Autodesk Inventor part; units mm, degrees
ref_plane "YZ Plane" through (0, 0, 0) normal (1, 0, 0) x (0, 1, 0)
ref_plane "XZ Plane" through (0, 0, 0) normal (0, 1, 0) x (-1, 0, 0)
ref_plane "XY Plane" through (0, 0, 0) normal (0, 0, 1) x (1, 0, 0)
sketch "Sketch1" plane through (0, 0, 0) normal (0, 1, 0) x (-1, 0, 0)
  circle A0 centre (0, 0) radius 50
  dimension "d0" = 100
extrude "Extrusion1" add sketch "Sketch1" along normal mid plane 5
sketch "Sketch2" plane through (0, 2.5, 0) normal (0, 1, 0) x (1, 0, 0)
  line L0 (-5, 5) -> (5, 5) construction
  line L1 (5, 5) -> (5, -5) construction
  line L2 (5, -5) -> (-5, -5) construction
  line L3 (-5, -5) -> (-5, 5) construction
  line L4 (-5, 5) -> (5, -5) construction
  line L5 (5, 5) -> (-5, -5) construction
  circle A0 centre (5, 5) radius 2.75
  circle A1 centre (-5, -5) radius 2.75
  point P0 (0, 0)
  dimension "d77" = 10
  dimension "d78" = 10
  dimension "d80" = 5.5
  dimension "d81" = 5.5
extrude "Extrusion2" cut sketch "Sketch2" against normal blind 10
sketch "Sketch3" plane through (0, 2.5, 0) normal (0, 1, 0) x (1, 0, 0)
  line L0 (0, 0) -> (25, 0) construction
  line L1 (18.8, -11.3) -> (31.2, -11.3)
  line L2 (31.2, -11.3) -> (31.2, 11.3)
  line L3 (31.2, 11.3) -> (18.8, 11.3)
  line L4 (18.8, 11.3) -> (18.8, -11.3)
  line L5 (18.8, -11.3) -> (31.2, 11.3) construction
  line L6 (31.2, -11.3) -> (18.8, 11.3) construction
  line L7 (25, 0) -> (25, 14.25) construction
  line L8 (25, 0) -> (25, -14.25) construction
  circle A0 centre (25, 14.25) radius 1.1
  circle A1 centre (25, -14.25) radius 1.1
  dimension "d9" = 25
  dimension "d10" = 12.4
  dimension "d11" = 22.6
  dimension "d21" = 14.25
  dimension "d22" = 14.25
  dimension "d23" = 2.2
  dimension "d24" = 2.2
extrude "Extrusion3" cut sketch "Sketch3" against normal blind 10
sketch "Sketch5" plane through (0, -2.5, 0) normal (0, -1, 0) x (1, 0, 0)
  line L0 (31.2, -11.3) -> (33.7, -11.3)
  line L1 (33.7, -11.3) -> (33.7, 11.3)
  line L2 (33.7, 11.3) -> (31.2, 11.3)
  line L3 (31.2, 11.3) -> (31.2, -11.3)
  line L4 (31.2, -11.3) -> (31.2, 11.3) construction
  line L5 (31.2, 0) -> (39.7, 0) construction
  line L6 (39.7, 0) -> (39.7, -20) construction
  line L7 (39.7, -20) -> (31.2, -20)
  line L8 (31.2, -20) -> (31.2, 20)
  line L9 (31.2, 20) -> (39.7, 20)
  line L10 (39.7, 20) -> (39.7, -20)
  line L11 (33.7, -11.3) -> (33.7, -20)
  line L12 (33.7, 11.3) -> (33.7, 20)
  point P0 (0, 0)
  point P1 (31.2, 11.3)
  dimension "d34" = 2.5
  dimension "d35" = 8.5
  dimension "d36" = 20
  dimension "d37" = 40
extrude "Extrusion5" add sketch "Sketch5" along normal blind 11.8 contours L1 L12 L9 L10 L7 L11
sketch "Sketch6" plane through (0, -2.5, 0) normal (0, -1, 0) x (1, 0, 0)
  line L0 (31.2, -11.3) -> (31.2, 11.3)
  line L1 (31.2, 0) -> (33.7, 0)
  line L2 (33.7, 0) -> (33.7, -20)
  line L3 (33.7, -20) -> (31.2, -20)
  line L4 (31.2, -20) -> (31.2, 0)
  line L5 (39.7, 20) -> (33.7, 20)
  line L6 (31.2, 0) -> (33.7, 0)
  line L7 (33.7, 0) -> (33.7, 20)
  line L8 (33.7, 20) -> (31.2, 20)
  line L9 (31.2, 20) -> (31.2, 0)
  line L10 (18.8, 11.3) -> (31.2, 11.3)
  line L11 (31.2, 11.3) -> (33.7, 11.3)
  line L12 (33.7, -20) -> (33.7, 20)
  line L13 (39.7, 20) -> (42.2, 20)
  line L14 (42.2, 20) -> (42.2, -20)
  line L15 (42.2, -20) -> (39.7, -20)
  line L16 (39.7, -20) -> (39.7, 20)
  line L17 (31.2, -15.9678) -> (33.7, -15.9678)
  point P0 (0, 0)
  point P1 (31.2, 11.3)
  dimension "d40" = 2.5
extrude "Extrusion6" add sketch "Sketch6" along normal blind 16.8 contours L13 L14 L15 L16 | L17 L2 L3 L4 | L9 L8 L7 L11
sketch "Sketch7" plane through (0, -19.3, 0) normal (0, -1, 0) x (1, 0, 0)
  line L0 (42.2, -20) -> (31.2, -20)
  line L1 (31.2, -20) -> (42.2, -20)
  line L2 (42.2, -20) -> (42.2, 0)
  line L3 (42.2, 0) -> (31.2, 0)
  line L4 (31.2, 0) -> (31.2, -20)
  point P0 (0, 0)
extrude "Extrusion7" add sketch "Sketch7" along normal blind 2.5
sketch "Sketch8" plane through (31.2, -19.3, 0) normal (0, 0, 1) x (1, 0, 0)
  line L0 (0, -2.5) -> (11, -2.5) construction
  line L1 (5.5, -2.5) -> (5.5, -10) construction
  circle A0 centre (5.5, -10) radius 7.5
  line L2 (0, 16.8) -> (0, -2.5) construction
  line L3 (11, 16.8) -> (11, -2.5)
  line L4 (11, -2.5) -> (11, -4.901)
  line L5 (0, -2.5) -> (0, -4.901)
  line L6 (11, -2.5) -> (0, -2.5)
  point P0 (-31.2, 19.3)
  dimension "d45" = 7.5
extrude "Extrusion8" add sketch "Sketch8" against normal blind 3
fillet "Fillet1" radius 8.25 1 edges at (36.7, -21.8, -3)
sketch "Sketch9" plane through (42.2, -2.5, -20) normal (0, 0, -1) x (-1, 0, 0)
  line L0 (11, -16.8) -> (8.5, -16.8)
  line L1 (8.5, -16.8) -> (2.5, -16.8)
  line L2 (2.5, -16.8) -> (2.5, -11.8)
  line L3 (2.5, -11.8) -> (8.5, -11.8)
  line L4 (8.5, -11.8) -> (8.5, -16.8)
  line L5 (11, 0) -> (11, -19.3)
  line L6 (0, 0) -> (0, -19.3)
  line L7 (11, -19.3) -> (0, -19.3)
  line L8 (0, -19.3) -> (0, -9.35)
  line L9 (0, -9.35) -> (11, -9.35)
  line L10 (11, -9.35) -> (11, -19.3)
  point P0 (42.2, 2.5)
  dimension "d49" = 9.95
extrude "Extrusion9" add sketch "Sketch9" along normal blind 10
sketch "Sketch12" plane through (0, 2.5, 0) normal (0, 1, 0) x (1, 0, 0)
  circle A0 centre (-25, 0) radius 12.5 construction
  line L0 (-25, 0) -> (-18.75, -10.8253) construction
  line L1 (-25, 0) -> (-37.5, 0) construction
  line L2 (-25, 0) -> (-18.75, 10.8253) construction
  circle A1 centre (-37.5, 0) radius 2.75
  circle A2 centre (-18.75, 10.8253) radius 2.75
  circle A3 centre (-18.75, -10.8253) radius 2.75
  point P0 (0, 0)
  dimension "d64" = 25
  dimension "d65" = 120
  dimension "d67" = 5.5
  dimension "d68" = 5.5
  dimension "d69" = 5.5
  dimension "d70" = 25
extrude "Extrusion12" cut sketch "Sketch12" against normal blind 10
sketch "Sketch13" plane through (0, -2.5, 0) normal (0, -1, 0) x (1, 0, 0)
  line L0 (0, 0) -> (0, -35) construction
  circle A0 centre (0, -35) radius 10.5
  dimension "d73" = 35
  dimension "d74" = 21
extrude "Extrusion13" cut sketch "Sketch13" against normal blind 10
sketch "Sketch14" plane through (31.2, -2.5, 20) normal (0, 0, 1) x (1, 0, 0)
  line L0 (8.5, -16.8) -> (2.5, -16.8)
  line L1 (2.5, -16.8) -> (2.5, -11.8)
  line L2 (2.5, -11.8) -> (8.5, -11.8)
  line L3 (8.5, -11.8) -> (8.5, -16.8)
  line L4 (1.5, -17.8) -> (9.5, -17.8)
  line L5 (9.5, -17.8) -> (9.5, -10.8)
  line L6 (9.5, -10.8) -> (1.5, -10.8)
  line L7 (1.5, -10.8) -> (1.5, -17.8)
  point P0 (-31.2, 2.5)
  dimension "d83" = 1
extrude "Extrusion14" cut sketch "Sketch14" against normal through all
sketch "Sketch17" plane through (0, -2.5, 0) normal (0, -1, 0) x (1, 0, 0)
  line L0 (0, 0) -> (0, 40) construction
  line L1 (-17, 40) -> (17, 40) construction
  line L2 (-17, 37.25) -> (17, 37.25)
  line L3 (17, 42.75) -> (-17, 42.75)
  arc A0 (-17, 42.75) -> (-17, 37.25) centre (-17, 40) ccw
  arc A1 (17, 37.25) -> (17, 42.75) centre (17, 40) ccw
  dimension "d104" = 17
  dimension "d105" = 5.5
extrude "Extrusion15" cut sketch "Sketch17" against normal through all
sketch "Sketch18" plane through (0, -2.5, 0) normal (0, -1, 0) x (1, 0, 0)
  line L0 (31.2, 20) -> (31.2, 11.3)
  line L1 (31.2, 11.3) -> (31.2, 12.3)
  line L2 (31.2, 12.3) -> (17.8, 12.3)
  line L3 (17.8, 12.3) -> (31.2, 12.3)
  line L4 (31.2, 12.3) -> (31.2, -12.3)
  line L5 (31.2, -12.3) -> (17.8, -12.3)
  line L6 (17.8, -12.3) -> (17.8, 12.3)
  point P0 (0, 0)
  dimension "d93" = 1
  dimension "d94" = 13.4
  dimension "d95" = 24.6
extrude "Extrusion16" cut sketch "Sketch18" against normal blind 10
sketch "Sketch19" plane through (31.2, -19.3, 11.3) normal (-1, 0, 0) x (0, 0, 1)
  line L0 (-27.2678, 6) -> (0, 6)
  line L1 (8.7, 0) -> (0, 0)
  line L2 (0, 6) -> (4.35, 6)
  line L3 (4.35, 6) -> (4.35, 0)
  line L4 (4.35, 0) -> (0, 0)
  line L5 (0, 0) -> (0, 6)
  point P0 (-11.3, 19.3)
extrude "Extrusion17" cut sketch "Sketch19" against normal up to surface (1.5 mm away)
sketch "Sketch22" plane through (0, 2.5, 0) normal (0, 1, 0) x (1, 0, 0)
  circle A0 centre (0, 35) radius 10.5
  line L0 (0, 35) -> (-20, 35) construction
  circle A1 centre (-20, 35) radius 2.75
  point P0 (0, 0)
  dimension "d100" = 20
  dimension "d101" = 5.5
extrude "Extrusion18" cut sketch "Sketch22" against normal blind 10 contours A1
equation "\"d80\" = d82"
equation "\"d81\" = d82"
properties part number "EndEffectorPlate" material "ABS Plastic"
Could you check a few things on this model? Use its own coordinates, in mm. A direction names the side the tool comes from. Round coordinates to 2 decimals unless told otherwise and drop trailing zeros. Loops run counter-clockwise (first coordinate to the right, second up) from the corner with the lowest first, then second, coordinate; pieces in that order, holes last. Notation, with made-up numbers: (6.5, -40) - (64.5, -40) arc R25 cw to (64.5, -23) - close; hole circle Ø4 at (81, -1). An arc over 180 degrees is marked (long way). Answer in a Markdown table with one row per item. Add a question column.
(1) I'm going to push flat-ended pins straight in: pin 1 (4 mm diameter, centred on x = 22.5, y = 0.5, fed in from -Z); pin 2 (1.2 mm diameter, centred on x = 41, z = 5.5, fed in from -Y); pin 3 (2 mm diameter, centred on y = -15.5, z = -19, fed in from +X). Where does each tip first touch, or does it pass through?
(2) If we section it at A-A (y = -18): Please give me the cut outline in (x, z).
(3) If we mould it in two halves opening along Z, with no side actions, what happens to faces 1 (the face through (37, -9, 20)), 2 (the face through (37, -11.85, -25)), 3 (the face through (17.8, 0, 0))? For each: pulls with the +Z half, pulls with the -Z half, needs draft (parallel to the pull), parting line crosses it, or undercut.
(4) I need wall thicknesses on line 1 along X through (y, z) = (-0.9, 5); line 2 along Z through (x, y) = (-5, 1); line 3 along X through (y, z) = (-19, -7). Which ranges of each line are inside material? Lowest first, please.
(5) If we section it at D-D (x = -38): Please give me the cut outline in (y, z), plus the area to 3 significant figures.
(6) If we section it at B-B (x = 0): Please give me the cut outline in (y, z), plus the area to 4 significant figures.
(7) For faces 4 (the face through (32.7, -16, 18)), 5 (the face through (42.2, -13, -5)), 6 (the face through (25, 0, 12.3)), which set-ups out of +Z, -Z, +X, -X, +Y, -Y let a thin tool reach every point of the face, with its end or its side?
(8) If we section it at C-C (y = -10.5): Please give me the cut outline in (x, z), plus the area to 3 significant figures.
Model answer:
| question | item | result |
|---|---|---|
| 1 | pin 1 | stops at z = -45.6 |
| 1 | pin 2 | stops at y = -19.3 |
| 1 | pin 3 | stops at x = 42.2 |
| 2 | outline | (31.2, -30) - (32.7, -30) - (32.7, -15.97) - (31.2, -15.97) - close; (31.2, 15.65) - (32.7, 15.65) - (32.7, 20) - (31.2, 20) - close; (40.7, -30) - (42.2, -30) - (42.2, 20) - (40.7, 20) - close |
| 3 | face 1 | pulls with the +Z half |
| 3 | face 2 | needs draft |
| 3 | face 3 | undercut |
| 4 | line 1 | x = -49.75 to -7.75, -2.25 to 17.8, 31.2 to 49.75 |
| 4 | line 2 | z = -49.75 to -44.23, -25.77 to 2.25, 7.75 to 37.25, 42.75 to 49.75 |
| 4 | line 3 | x = 40.7 to 42.2 |
| 5 | outline | (-2.5, -32.5) - (2.5, -32.5) - (2.5, -2.7) - (-2.5, -2.7) - close; (-2.5, 2.7) - (2.5, 2.7) - (2.5, 32.5) - (-2.5, 32.5) - close |
| 5 | area | 298 mm² |
| 6 | outline | (-2.5, -50) - (2.5, -50) - (2.5, -45.5) - (-2.5, -45.5) - close; (-2.5, -24.5) - (2.5, -24.5) - (2.5, 37.25) - (-2.5, 37.25) - close; (-2.5, 42.75) - (2.5, 42.75) - (2.5, 50) - (-2.5, 50) - close |
| 6 | area | 367.5 mm² |
| 7 | face 4 | +Z, -Z, -Y |
| 7 | face 5 | +Z, -Z, +X |
| 7 | face 6 | +Y, -Y |
| 8 | outline | (31.2, -20) - (42.2, -20) - (42.2, 20) - (31.2, 20) - (31.2, 11.3) - (33.7, 11.3) - (33.7, -15.97) - (31.2, -15.97) - close |
| 8 | area | 372 mm² |
